```python
from build123d import *

# Parameters (mm, degrees)
F1_DEPTH      = 30
F1_DEPTH_BACK = 225
F2_DEPTH      = 2


with BuildPart() as f1:
    # F0 (on Top) → F1 (new body, two sides)
    with BuildSketch(Plane.XY) as f1_sk:
        with BuildLine():
            Line((0, -9.9217584357), (0, 10.0142153224))
            ThreePointArc((0, 10.0142153224), (-7.0811195627, 7.0811195627), (-10.0142153224, 0))
            ThreePointArc((-10.0142153224, 0), (-7.5458705502, -6.5836423174), (-1.3576516741, -9.9217584357))
            Line((-1.3576516741, -9.9217584357), (0, -9.9217584357))
        make_face()
        with BuildLine():
            ThreePointArc((1.3576516741, -9.9217584357), (7.5458705502, -6.5836423174), (10.0142153224, 0))
            ThreePointArc((10.0142153224, 0), (7.0811195627, 7.0811195627), (0, 10.0142153224))
            Line((0, 10.0142153224), (0, -9.9217584357))
            Line((0, -9.9217584357), (1.3576516741, -9.9217584357))
        make_face()
    extrude(amount=F1_DEPTH)
    extrude(f1_sk.sketch, amount=-F1_DEPTH_BACK)

    # F0 (on Top) → F2 (join)
    with BuildSketch(Plane.XY):
        with BuildLine():
            Line((10.0142153224, -9.9217584357), (1.3576516741, -9.9217584357))
            ThreePointArc((1.3576516741, -9.9217584357), (0, -10.0142153224), (-1.3576516741, -9.9217584357))
            Line((-1.3576516741, -9.9217584357), (-10.0142153224, -9.9217584357))
            Line((-10.0142153224, -9.9217584357), (-10.0142153224, -147.4426090717))
            Line((-10.0142153224, -147.4426090717), (10.0142153224, -147.4426090717))
            Line((10.0142153224, -147.4426090717), (10.0142153224, -9.9217584357))
        make_face()
        with BuildLine():
            ThreePointArc((-10.0142153224, -147.4426090717), (0, -157.4568243942), (10.0142153224, -147.4426090717))
            Line((10.0142153224, -147.4426090717), (-10.0142153224, -147.4426090717))
        make_face()
        with BuildLine():
            ThreePointArc((147.6441994309, -9.9217584357), (157.61218631, 0.0462284434), (147.6441994309, 10.0142153224))
            Line((147.6441994309, 10.0142153224), (147.6441994309, -9.9217584357))
        make_face()
        Polygon((10.0142153224, 10.0142153224), (10.0142153224, 0), (10.0142153224, -9.9217584357), (147.6441994309, -9.9217584357), (147.6441994309, 10.0142153224), align=None)
        Polygon((-10.0142153224, -9.9217584357), (-10.0142153224, 0), (-10.0142153224, 10.0142153224), (-147.6441994309, 10.0142153224), (-147.6441994309, -9.9217584357), align=None)
        Polygon((-10.0142153224, 10.0142153224), (0, 10.0142153224), (10.0142153224, 10.0142153224), (10.0142153224, 147.4426090717), (-10.0142153224, 147.4426090717), align=None)
        with BuildLine():
            Line((-10.0142153224, 147.4426090717), (10.0142153224, 147.4426090717))
            ThreePointArc((10.0142153224, 147.4426090717), (0, 157.4568243942), (-10.0142153224, 147.4426090717))
        make_face()
        with BuildLine():
            Line((-147.6441994309, -9.9217584357), (-147.6441994309, 10.0142153224))
            ThreePointArc((-147.6441994309, 10.0142153224), (-157.61218631, 0.0462284434), (-147.6441994309, -9.9217584357))
        make_face()
        with BuildLine():
            ThreePointArc((0, 10.0142153224), (7.0811195627, 7.0811195627), (10.0142153224, 0))
            Line((10.0142153224, 0), (10.0142153224, 10.0142153224))
            Line((10.0142153224, 10.0142153224), (0, 10.0142153224))
        make_face()
        with BuildLine():
            ThreePointArc((-10.0142153224, 0), (-7.0811195627, 7.0811195627), (0, 10.0142153224))
            Line((0, 10.0142153224), (-10.0142153224, 10.0142153224))
            Line((-10.0142153224, 10.0142153224), (-10.0142153224, 0))
        make_face()
        with BuildLine():
            ThreePointArc((-1.3576516741, -9.9217584357), (-7.5458705502, -6.5836423174), (-10.0142153224, 0))
            Line((-10.0142153224, 0), (-10.0142153224, -9.9217584357))
            Line((-10.0142153224, -9.9217584357), (-1.3576516741, -9.9217584357))
        make_face()
        with BuildLine():
            Line((10.0142153224, -9.9217584357), (10.0142153224, 0))
            ThreePointArc((10.0142153224, 0), (7.5458705502, -6.5836423174), (1.3576516741, -9.9217584357))
            Line((1.3576516741, -9.9217584357), (10.0142153224, -9.9217584357))
        make_face()
    extrude(amount=F2_DEPTH)

    # F3 (on Front) → F4 (revolve)
    with BuildSketch(Plane.XZ):
        Polygon((0, -265.1076316833), (0, -224.9582111835), (-10.0062908605, -224.9979376793), align=None)
        with BuildLine():
            ThreePointArc((-10.0062908605, -224.9979376793), (-6.1254784251, -245.3327766052), (0, -265.1076316833))
            Line((0, -265.1076316833), (-10.0062908605, -224.9979376793))
        make_face()
    revolve(axis=Axis((0, 0, -245.0329214334), (0, 0, -1)))


solid = f1.part
```
Model file for the job. Use its own axes, mm. A direction names the side the tool comes from. Coordinates: 2 decimals unless noted, no trailing zeros. Loops run counter-clockwise (first coordinate to the right, second up) from the corner with the lowest first, then second, coordinate; pieces in that order, holes last. Notation, with made-up numbers: M 57,-17.5 L 105,-17.5 A9 cw 105,-13.5 Z; hole C 38.5,-5.5 d10. An arc over 180 degrees is marked long. Use CSV: the item, a comma, the result in double quotes. Start each with the question number.
1. Band-saw the part on B-B, the plane y = 138. List the corners of the cut face in (x, z).
2. Band-saw the part on A-A, the plane z = -92.5. List the corners of the cut face in (x, y).
3. Probe probe 1 along X at (y, z) = (-33, 1.5); probe 2 along Z at (x, y) = (0.5, 127). List the from-to ranges inside material, lowest first. Write a range as [from, to].
4. Band-saw the part on C-C, the plane x = -112.5. List the corners of the cut face in (y, z), then the cut area to 3 significant figures.
5. Flat gauge pins, fed straight in: pin 1 (2 mm diameter, centred on x = -96, z = 1, fed in from +Y); pin 2 (1.6 mm diameter, centred on y = -45, z = 1, fed in from +X); pin 3 (1 mm diameter, centred on x = 51.5, z = 1, fed in from -Y). Where does each tip first touch, or does it go through?
6. Tool access for faces 1 (the cylindrical face through (0.22, 157.454, 0.986)), 2 (the flat face through (-1, -11, 0)), 3 (the flat face through (-1, -11, 2)): list every direction of +Z, -Z, +X, -X, +Y, -Y with a clear straight run to the whole face (end or side of a thin tool).
Entries:
1,outline,"M -10.01,0 L 10.01,0 L 10.01,2 L -10.01,2 Z"
2,outline,"M -1.36,-9.92 L 1.36,-9.92 A10.01 ccw long Z"
3,probe 1,"x = [-10.01, 10.01]"
3,probe 2,"z = [0, 2]"
4,outline,"M -9.92,0 L 10.01,0 L 10.01,2 L -9.92,2 Z"
4,area,"39.9 mm2"
5,pin 1,"stops at y = 10.01"
5,pin 2,"stops at x = 10.01"
5,pin 3,"stops at y = -9.92"
6,face 1,"+Z, -Z, +Y"
6,face 2,"-Z"
6,face 3,"+Z"
